Geometry check sheet. Reference: the model listing, model coordinates, mm. A direction names the side the tool comes from. Round coordinates to 2 decimals unless told otherwise and drop trailing zeros. Write each loop counter-clockwise with the first axis right and the second up, starting at its lowest first coordinate (ties: lowest second). Pieces come first, ordered by that corner, then holes. Notation, with made-up numbers: M -8.75,26 L 28.25,26 A20 ccw 28.25,65 Z; hole C 58.25,13 d7. An arc over 180 degrees is marked long. Use a Markdown table: item, result.
Autodesk Inventor part; units mm, degrees
ref_plane "YZ Plane" through (0, 0, 0) normal (1, 0, 0) x (0, 1, 0)
ref_plane "XZ Plane" through (0, 0, 0) normal (0, 1, 0) x (-1, 0, 0)
ref_plane "XY Plane" through (0, 0, 0) normal (0, 0, 1) x (1, 0, 0)
sketch "Skizze1" plane through (0, 0, 0) normal (0, 1, 0) x (-1, 0, 0)
  line L0 (0, 0) -> (30, 0)
  line L1 (30, 0) -> (30, -16)
  line L2 (30, -16) -> (0, -16)
  line L3 (0, -16) -> (0, 0)
  dimension "d0" = 30
  dimension "d1" = 16
extrude "Extrusion1" add sketch "Skizze1" along normal blind 1
sketch "Skizze2" plane through (-30, 0, 0) normal (0, 0, 1) x (1, 0, 0)
  line L0 (30, 1) -> (0, 1)
  line L1 (27.5, 1) -> (27.5, 14.5)
  line L2 (27.5, 1) -> (41, 1) construction
  line L3 (27.5, 14.5) -> (25.5, 14.5)
  line L4 (25.5, 14.5) -> (25.5, 13.5)
  line L5 (25.5, 13.5) -> (26.5, 13.5)
  line L6 (26.5, 13.5) -> (26.5, 1)
  line L7 (26.5, 1) -> (27.5, 1)
  line L8 (15, 1) -> (15, 5.7863)
  point P0 (30, 0)
  point P1 (15, 3.3931)
  point P2 (26.5, 1)
  dimension "d4" = 13.5
  dimension "d5" = 90
  dimension "d6" = 2
  dimension "d7" = 1
  dimension "d8" = 1
  dimension "d9" = 11.5
extrude "Extrusion2" add sketch "Skizze2" against normal blind 16
ref_plane "Arbeitsebene1" through (-15, 0, 0) normal (1, 0, 0) x (0, 0, -1)
sketch "Skizze3" plane through (-2.5, 1, 0) normal (1, 0, 0) x (0, 0, -1)
  line L0 (16, 0) -> (0, 0)
  line L1 (4, 0) -> (7, 0)
  line L2 (7, 0) -> (7, 14.6067)
  line L3 (7, 14.6067) -> (4, 14.6067)
  line L4 (4, 14.6067) -> (4, 0)
  point P0 (0, -1)
  point P1 (7, 0)
  dimension "d12" = 3
extrude "Extrusion3" cut sketch "Skizze3" against normal blind 16
mirror "Spiegeln1" about plane through (-15, 0, 0) normal (1, 0, 0) of "Extrusion2", "Extrusion3"
equation "\"Biegeradius\" = Stärke"
equation "\"BreiteBiegungsfreistellung\" = Stärke"
equation "\"TiefeBiegungsfreistellung\" = 0.5 * Stärke"
equation "\"GrößeEckenfreistellung\" = 4 * Stärke"
equation "\"MinimalRest\" = 2 * Stärke"
equation "\"Übergangsradius\" = Biegeradius"
equation "\"JacobiRadiusGröße\" = Biegeradius"
equation "\"Abstandsgröße\" = Stärke"
properties part number "ServoHalterung"
Item 1: Access from +Z, -Z, +X, -X, +Y, -Y to the whole of each face (thin tool, end or side, straight path). Record for faces 4 (the face through (-2.5, 8, -11)), 5 (the face through (-26.5, 7, -2)), 6 (the face through (-27, 8, -4)), 7 (the face through (-25.5, 14, -11)).
Outcome:
| item | result |
|---|---|
| face 4 | +Z, -Z, +X, +Y |
| face 5 | +Z, -Z |
| face 6 | +X, -X, +Y |
| face 7 | +Z, -Z, +Y |
Item 2: Cross-section at B-B, the plane z = -14. Record the cut outline in (x, y).
Outcome:
| item | result |
|---|---|
| outline | M -30,0 L 0,0 L 0,1 L -2.5,1 L -2.5,14.5 L -4.5,14.5 L -4.5,13.5 L -3.5,13.5 L -3.5,1 L -26.5,1 L -26.5,13.5 L -25.5,13.5 L -25.5,14.5 L -27.5,14.5 L -27.5,1 L -30,1 Z |
Item 3: Cross-section at C-C, the plane x = -11. Record the cut outline in (y, z).
Outcome:
| item | result |
|---|---|
| outline | M 0,-16 L 1,-16 L 1,0 L 0,0 Z |
Item 4: Cross-section at A-A, the plane y = 3. Record the cut outline in (x, z), and give its area (3 significant figures).
Outcome:
| item | result |
|---|---|
| outline | M -27.5,-16 L -26.5,-16 L -26.5,-7 L -27.5,-7 Z; M -27.5,-4 L -26.5,-4 L -26.5,0 L -27.5,0 Z; M -3.5,-16 L -2.5,-16 L -2.5,-7 L -3.5,-7 Z; M -3.5,-4 L -2.5,-4 L -2.5,0 L -3.5,0 Z |
| area | 26.0 mm2 |
Item 5: Material ranges on line 1 along X through (y, z) = (5.25, -14.25); line 2 along Y through (x, z) = (-25.75, -15); line 3 along Y through (x, z) = (-6.75, -5.25), recorded low to high. Write a range as from..to.
Outcome:
| item | result |
|---|---|
| line 1 | x = -27.5..-26.5, -3.5..-2.5 |
| line 2 | y = 0..1, 13.5..14.5 |
| line 3 | y = 0..1 |
Item 6: Cross-section at D-D, the plane z = -6.25. Record the cut outline in (x, y), and give its area (3 significant figures).
Outcome:
| item | result |
|---|---|
| outline | M -30,0 L 0,0 L 0,1 L -30,1 Z |
| area | 30.0 mm2 |
Item 7: Go/stop test with flat-tipped pins: pin 1 (1.1 mm diameter, centred on y = 14, z = -1, fed in from -X); pin 2 (1.2 mm diameter, centred on y = 6.5, z = -3, fed in from +X); pin 3 (8 mm diameter, centred on x = -8.5, z = -6, fed in from +Y). Record where each tip stops, or that it passes through.
Outcome:
| item | result |
|---|---|
| pin 1 | stops at x = -27.5 |
| pin 2 | stops at x = -2.5 |
| pin 3 | stops at y = 1 |
Item 8: Mould release check, pull along X, two halves, no side actions. Record for faces 1 (the face through (-15, 0, -8)), 2 (the face through (-4.5, 14, -2)), 3 (the face through (0, 0.5, -8.1)): +X half, -X half, draft (parallel to the pull), parting line (faces both ways), or undercut.
Outcome:
| item | result |
|---|---|
| face 1 | draft |
| face 2 | undercut |
| face 3 | +X half |
